Read the model definition and answer for the solid it produces. Units are mm, in the model's axes. Face numbers are marked on the shaded views. Give positions to 0.01 mm unless a question says otherwise; leave off trailing zeros. Order: outer loops, then holes, each group sorted by start corner. A loop starts at its lowest first (then second) coordinate and runs counter-clockwise, first axis right, second up. Notation, with made-up numbers: (-34, 66.5) - (-25, 66.5) arc R35 ccw to (-25, 98.5) - close; hole circle Ø2 at (-10.5, 87). An arc over 180 degrees is marked (long way). Use a Markdown table: item, result. Add a question column.
1. A cutting plane is placed at C-C on y = 29. Determine the outline of the cut face in (x, z) (3 decimals).
2. A flat-ended cylindrical pin translates along its axis: P1, Ø4.5, axis at x = 0, z = 0, coming from the +Y side. Find the tip coordinate at first contact, or state that the pin passes through.
3. A cutting plane is placed at A-A on x = 0. Determine the outline of the cut face in (y, z) (3 decimals).
4. Consider L1, parallel to Z at x = 0, y = 21 (3 decimals); L2, parallel to Z at x = 1.75, y = 3 (3 decimals). Determine where each line is inside the solid, lowest interval first.
5. A cutting plane is placed at B-B on z = -1.5. Determine the outline of the cut face in (x, y) (3 decimals).
6. For a pull along Z with two mould halves and no side action, classify the marked faces 1, 2 and 3 as released by +Z, released by -Z, zero draft, split by the parting line, or undercut.
```python
from build123d import *

# Parameters (mm, degrees)
SKETCH_2_W      = 27.85
SKETCH_2_H      = 27.85
SKETCH_2_R      = 2.5
EXTRUDE_1_DEPTH = 36
CHAMFER_1_SIZE  = 2


with BuildPart() as part:
    # Эскиз2 → Бобышка-Вытянуть1 (new body)
    with BuildSketch(Plane(origin=(0, 0, 0), x_dir=(1, 0, 0), z_dir=(0, 1, 0))):
        Rectangle(SKETCH_2_W, SKETCH_2_H)
        Circle(SKETCH_2_R, mode=Mode.SUBTRACT)
    extrude(amount=EXTRUDE_1_DEPTH)

    # Фаска1
    chamfer_1_edges = [part.edges().sort_by_distance(p)[0] for p in [
        (13.925, 18, -13.925),
        (13.925, 18, 13.925),
        (-13.925, 18, 13.925),
        (-13.925, 18, -13.925),
    ]]
    chamfer(chamfer_1_edges, length=CHAMFER_1_SIZE)


solid = part.part
```
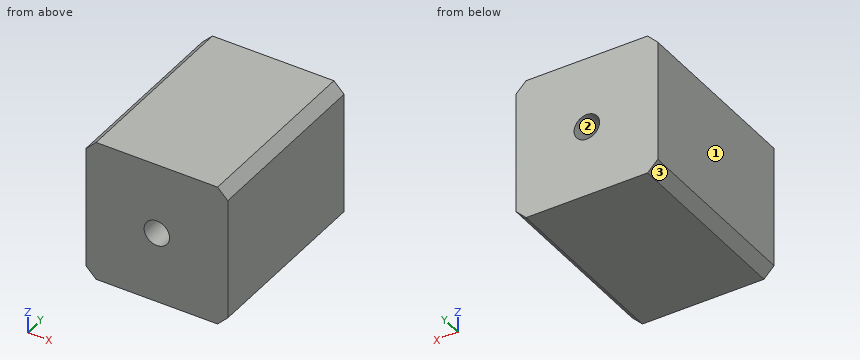
Output values:
| question | item | result |
|---|---|---|
| 1 | outline | (-13.925, -11.925) - (-11.925, -13.925) - (11.925, -13.925) - (13.925, -11.925) - (13.925, 11.925) - (11.925, 13.925) - (-11.925, 13.925) - (-13.925, 11.925) - close; hole circle Ø5 at (0, 0) |
| 2 | P1 | through |
| 3 | outline | (0, -13.925) - (36, -13.925) - (36, -2.5) - (0, -2.5) - close; (0, 2.5) - (36, 2.5) - (36, 13.925) - (0, 13.925) - close |
| 4 | L1 | -13.925 to -2.5, 2.5 to 13.925 |
| 4 | L2 | -13.925 to -1.785, 1.785 to 13.925 |
| 5 | outline | (-13.925, 0) - (-2, 0) - (-2, 36) - (-13.925, 36) - close; (2, 0) - (13.925, 0) - (13.925, 36) - (2, 36) - close |
| 6 | face 1 | zero draft |
| 6 | face 2 | undercut |
| 6 | face 3 | released by -Z |
